```python
from build123d import *

# Parameters (mm, degrees)
F0_R     = 39.5
F0_R_2   = 35
F1_DEPTH = 5
F0_R_3   = 43
F0_R_4   = 15
F2_DEPTH = 5
F3_R     = 4.99999
F4_SIZE  = 1


# Not quite as in the source:
# - a fillet or chamfer is up to 0.001 mm smaller than in the source, because OpenCascade refuses the exact size


with BuildPart() as f1:
    # F0 (on Top) → F1 (new body)
    with BuildSketch(Plane.XY):
        Circle(F0_R)
        Circle(F0_R_2, mode=Mode.SUBTRACT)
    extrude(amount=F1_DEPTH)

    # F0 (on Top) → F2 (join)
    with BuildSketch(Plane.XY):
        Circle(F0_R_3)
        Circle(F0_R, mode=Mode.SUBTRACT)
        Circle(F0_R)
        Circle(F0_R_2, mode=Mode.SUBTRACT)
        Circle(F0_R_2)
        Circle(F0_R_4, mode=Mode.SUBTRACT)
    extrude(amount=-F2_DEPTH)

    # F3 (radius 5 in the source; OpenCascade refuses exactly that, so slightly less here)
    f3_edges = [f1.edges().sort_by_distance(p)[0] for p in [
        (-43, 0, -5),
    ]]
    fillet(f3_edges, radius=F3_R)

    # F4
    f4_edges = [f1.edges().sort_by_distance(p)[0] for p in [
        (-39.5, 0, 5),
    ]]
    chamfer(f4_edges, length=F4_SIZE)


solid = f1.part
```
Model file for the job. Use its own axes, mm. A direction names the side the tool comes from. Round coordinates to 2 decimals unless told otherwise and drop trailing zeros. Loops run counter-clockwise (first coordinate to the right, second up) from the corner with the lowest first, then second, coordinate; pieces in that order, holes last. Notation, with made-up numbers: M 33,45.25 L 50,45.25 A22 ccw 50,72.25 Z; hole C -35,44 d6. An arc over 180 degrees is marked long. Put each result on its own line as item: value. Start each with the question number.
Item 1: Cut at D-D (z = -3.75). List the corners of the cut face in (x, y).
Item 2: Drill centre lines: line 1 along Y through (x, z) = (0, 3.9); line 2 along Y through (x, z) = (0, -2.2); line 3 along Z through (x, y) = (-31, 22.5). Where is each one in solid material? Low to high.
Item 3: Drop flat-ended pins along their axis: P1, Ø1.5, axis at x = 34, z = 3, coming from the -Y side; P2, Ø1.5, axis at x = 18, z = 1.5, coming from the -Y side; P3, Ø21, axis at x = 2.5, y = -5, coming from the +Z side. Give the stop position or say it passes through.
Item 4: 3-axis set-ups, long thin cutter, end or side, ignore diameter. For faces 4 (the face through (15, -7, 0)), 5 (the face through (-14.985, 0.66, -2.465)): which of +Z, -Z, +X, -X, +Y, -Y reach the whole face in a straight line?
Item 5: Cut at C-C (z = 1.5). List the corners of the cut face in (x, y), then the cut area to 3 significant figures.
Item 6: Mould opens along X. For faces 1 (the face through (-29.11, 26.7, 1.97)), 2 (the face through (-28, -21, 2)), 3 (the face through (19, -35, 0)) say: released by +X, released by -X, zero draft, split by the parting line, or undercut.
Answer block:
1. outline: C 0,0 d82.61; hole C 0,0 d30
2. line 1: -39.5 to -35, 35 to 39.5
2. line 2: -42.49 to -15, 15 to 42.49
2. line 3: -4.99 to 5
3. P1: y = -21.32
3. P2: y = -35.53
3. P3: z = 0
4. face 4: +Z
4. face 5: +Z, -Z
5. outline: C 0,0 d79; hole C 0,0 d70
5. area: 1,050 mm2
6. face 1: split by the parting line
6. face 2: undercut
6. face 3: zero draft
